```python
from build123d import *

# Parameters (mm, degrees)
SKETCH1_R             = 33.3375
BOSS_EXTRUDE1_DEPTH   = 12.7
FILLET1_R             = 10
M5_TAPPED_HOLE1_D     = 4.2
M5_TAPPED_HOLE1_DEPTH = 14
M5_TAPPED_HOLE1_TIP   = 1.2618073
M6_TAPPED_HOLE1_D     = 5
M6_TAPPED_HOLE2_D     = 5
M6_TAPPED_HOLE3_D     = 5
M6_TAPPED_HOLE4_D     = 5
M6_TAPPED_HOLE5_D     = 5
M8_TAPPED_HOLE1_D     = 6.8
M6_TAPPED_HOLE6_D     = 5


with BuildPart() as part:
    # Sketch1 → Boss-Extrude1 (new body)
    with BuildSketch(Plane(origin=(0, 0, 0), x_dir=(0, 0, -1), z_dir=(1, 0, 0))):
        Polygon((26.5, 317.5), (262.5, 317.5), (262.5, -317.5), (-262.5, -317.5), (-262.5, 232.5), (26.5, 232.5), align=None)
        with Locations((82.5, 157.5)):
            Circle(SKETCH1_R, mode=Mode.SUBTRACT)
    extrude(amount=BOSS_EXTRUDE1_DEPTH)

    # Fillet1
    fillet1_edges = [part.edges().sort_by_distance(p)[0] for p in [
        (6.35, -317.5, -262.5),
        (6.35, -317.5, 262.5),
        (6.35, 232.5, 262.5),
        (6.35, 232.5, -26.5),
        (6.35, 317.5, -26.5),
        (6.35, 317.5, -262.5),
    ]]
    fillet(fillet1_edges, radius=FILLET1_R)

    # M5 Tapped Hole1
    with Locations(Plane(origin=(12.7, 0, 0), x_dir=(0, 0, -1), z_dir=(1, 0, 0))):
        with Locations((175.625, 302.5), (175.625, 280), (61.625, 280), (61.625, 302.5)):
            Hole(M5_TAPPED_HOLE1_D / 2, depth=M5_TAPPED_HOLE1_DEPTH)
            with Locations((0, 0, -(M5_TAPPED_HOLE1_DEPTH + M5_TAPPED_HOLE1_TIP / 2))):  # 118° drill point
                Cone(0, M5_TAPPED_HOLE1_D / 2, M5_TAPPED_HOLE1_TIP, mode=Mode.SUBTRACT)

    # M6 Tapped Hole1 (through all)
    with Locations(Plane(origin=(12.7, 0, 0), x_dir=(0, 0, -1), z_dir=(1, 0, 0))):
        with Locations((-186.587628, 5.81216), (-186.587628, -24.18784), (133.412372, 5.81216), (133.412372, -24.18784)):
            Hole(M6_TAPPED_HOLE1_D / 2)

    # M6 Tapped Hole2 (through all)
    with Locations(Plane(origin=(12.7, 0, 0), x_dir=(0, 0, -1), z_dir=(1, 0, 0))):
        with Locations((-210.013308, 42.88784), (-0.013308, 42.88784)):
            Hole(M6_TAPPED_HOLE2_D / 2)

    # M6 Tapped Hole3 (through all)
    with Locations(Plane(origin=(12.7, 0, 0), x_dir=(0, 0, -1), z_dir=(1, 0, 0))):
        with Locations((88.625, 220), (148.625, 220), (118.625, 100)):
            Hole(M6_TAPPED_HOLE3_D / 2)

    # M6 Tapped Hole4 (through all)
    with Locations(Plane(origin=(12.7, 0, 0), x_dir=(0, 0, -1), z_dir=(1, 0, 0))):
        with Locations((198.625, 292.5), (38.625, 292.5), (38.625, 52.5), (198.625, 52.5)):
            Hole(M6_TAPPED_HOLE4_D / 2)

    # M6 Tapped Hole5 (through all)
    with Locations(Plane(origin=(12.7, 0, 0), x_dir=(0, 0, -1), z_dir=(1, 0, 0))):
        with Locations((-14.1, -254.9), (-14.1, -88.9), (160.9, -297.4), (160.9, -88.9), (-14.1, -297.4)):
            Hole(M6_TAPPED_HOLE5_D / 2)

    # M8 Tapped Hole1 (through all)
    with Locations(Plane(origin=(12.7, 0, 0), x_dir=(0, 0, -1), z_dir=(1, 0, 0))):
        with Locations((-203.2135, -237.075), (-114.1865, -237.075), (-114.1865, -297.4), (-203.2135, -297.4)):
            Hole(M8_TAPPED_HOLE1_D / 2)

    # M6 Tapped Hole6 (through all)
    with Locations(Plane(origin=(12.7, 0, 0), x_dir=(0, 0, -1), z_dir=(1, 0, 0))):
        with Locations((-159.5, 220), (-95.5, 220), (-95.5, 132), (-159.5, 132)):
            Hole(M6_TAPPED_HOLE6_D / 2)


solid = part.part
```
The model under review builds one solid part; all positions refer to its coordinate system, in mm. A direction names the side the tool comes from. Round coordinates to 2 decimals unless told otherwise and drop trailing zeros. Loops run counter-clockwise (first coordinate to the right, second up) from the corner with the lowest first, then second, coordinate; pieces in that order, holes last. Notation, with made-up numbers: (60, 79.5) -> (81, 79.5) arc R21 ccw to (81, 109.5) -> close; hole circle Ø5 at (61.25, -37.5). An arc over 180 degrees is marked (long way). Answer in a Markdown table with one row per item.
1) Consider section C-C, the plane x = 4.25. Count the separate pieces of the cut face and the enclosed holes in it, plus the area to 3 significant figures.
Taken from the geometry:
| item | result |
|---|---|
| separate pieces | 1 |
| enclosed holes | 31 |
| area | 305,000 mm² |
2) For pin 1 Ø4.5 at (y, z) = (220, -88.625) entering from -X; pin 2 Ø6.5 at (y, z) = (280, -175.625) entering from +X; pin 3 Ø2 at (x, z) = (6.5, 50) entering from +Y, all flat-tipped, find the tip position at first contact; note any pin that passes through.
Taken from the geometry:
| item | result |
|---|---|
| pin 1 | passes through |
| pin 2 | stops at x = 12.7 |
| pin 3 | stops at y = 232.5 |
3) Consider section A-A, the plane y = 157.5. Write out the cut boundary in (x, z).
Taken from the geometry:
| item | result |
|---|---|
| outline | (0, -262.5) -> (12.7, -262.5) -> (12.7, -115.84) -> (0, -115.84) -> close; (0, -49.16) -> (12.7, -49.16) -> (12.7, 262.5) -> (0, 262.5) -> close |
4) Consider section B-B, the plane z = 48. Write out the cut boundary in (x, y), plus the area to 4 significant figures.
Taken from the geometry:
| item | result |
|---|---|
| outline | (0, -317.5) -> (12.7, -317.5) -> (12.7, 232.5) -> (0, 232.5) -> close |
| area | 6,985 mm² |
5) Wall thickness on line 1 along Y through (x, z) = (10.25, 159.5); line 2 along Z through (x, y) = (8, 220) (3 decimals); line 3 along Y through (x, z) = (5.25, 14.1): over which ranges is each line inside the solid? List them lowest first.
Taken from the geometry:
| item | result |
|---|---|
| line 1 | y = -317.5 to 129.5, 134.5 to 217.5, 222.5 to 232.5 |
| line 2 | z = -262.5 to -151.125, -146.125 to -91.125, -86.125 to 93, 98 to 157, 162 to 262.5 |
| line 3 | y = -317.5 to -299.9, -294.9 to -257.4, -252.4 to -91.4, -86.4 to 232.5 |
6) Tool access review of faces 1 (the flat face through (0, 4, -4)), 2 (the flat face through (6, 232.5, 120)): name each direction out of +Z, -Z, +X, -X, +Y, -Y from which nothing blocks a thin tool from reaching the whole face with its end or side.
Taken from the geometry:
| item | result |
|---|---|
| face 1 | +Z, -Z, -X, +Y, -Y |
| face 2 | +Z, +X, -X, +Y |
